Model file for the job. Use its own axes, mm. A direction names the side the tool comes from. Give positions to 0.01 mm unless a question says otherwise; leave off trailing zeros. Order: outer loops, then holes, each group sorted by start corner. A loop starts at its lowest first (then second) coordinate and runs counter-clockwise, first axis right, second up. Notation, with made-up numbers: (-27, 3) - (-17, 3) arc R35 ccw to (-17, 35) - close; hole circle Ø8 at (41, 14). An arc over 180 degrees is marked (long way). Return JSON: item names as keys, results as strings. Group by question number.
Autodesk Inventor part; units mm, degrees
ref_plane "YZ Plane" through (0, 0, 0) normal (1, 0, 0) x (0, 1, 0)
ref_plane "XZ Plane" through (0, 0, 0) normal (0, 1, 0) x (-1, 0, 0)
ref_plane "XY Plane" through (0, 0, 0) normal (0, 0, 1) x (1, 0, 0)
sketch "Sketch1" plane through (0, 0, 0) normal (0, 0, 1) x (1, 0, 0)
  circle A0 centre (0, 0) radius 12.5
  circle A1 centre (0, 0) radius 14.5
  dimension "d0" = 25
  dimension "d1" = 2
extrude "Extrusion1" add sketch "Sketch1" along normal blind 2
sketch "Sketch2" plane through (0, 0, 2) normal (0, 0, 1) x (1, 0, 0)
  circle A0 centre (0, 0) radius 14.5 construction
  line L0 (0, 14.5) -> (0, 0) construction
  line L1 (0, 0) -> (12.5574, -7.25) construction
  line L2 (0, 0) -> (-12.5574, -7.25) construction
  line L3 (0, 0) -> (-12.5574, 7.25) construction
  line L4 (0, 0) -> (12.5574, 7.25) construction
  circle A1 centre (0, 0) radius 14.5
  circle A2 centre (0, 0) radius 12.5
  line L5 (1.3066, 12.4315) -> (1.5157, 14.4206)
  line L6 (-1.3066, 12.4315) -> (-1.5157, 14.4206)
  line L7 (-11.4193, -5.0842) -> (-13.2464, -5.8977)
  line L8 (-10.1127, -7.3473) -> (-11.7307, -8.5229)
  line L9 (10.1127, -7.3473) -> (11.7307, -8.5229)
  line L10 (11.4193, -5.0842) -> (13.2464, -5.8977)
  line L11 (10.1127, 7.3473) -> (11.7307, 8.5229)
  line L12 (11.4193, 5.0842) -> (13.2464, 5.8977)
  line L13 (-11.4193, 5.0842) -> (-13.2464, 5.8977)
  line L14 (-10.1127, 7.3473) -> (-11.7307, 8.5229)
  line L15 (1.3066, -12.4315) -> (1.5157, -14.4206)
  line L16 (-1.3066, -12.4315) -> (-1.5157, -14.4206)
  point P0 (-12.5574, -7.25)
  point P1 (12.5574, -7.25)
  dimension "d4" = 120
  dimension "d5" = 120
  dimension "d6" = 6
  dimension "d7" = 6
  dimension "d10" = 360
  dimension "d14" = 6
  dimension "d15" = 6
  dimension "d18" = 360
extrude "Extrusion2" add sketch "Sketch2" along normal blind 16 contours A1 L9 A2 L10 | L5 A2 L6 A1 | A1 L7 A2 L8
sketch "Sketch3" plane through (0, 0, 2) normal (0, 0, 1) x (1, 0, 0)
  circle A0 centre (0, 0) radius 14.5 construction
  line L0 (0, 14.5) -> (0, 0) construction
  line L1 (0, 0) -> (12.5574, -7.25) construction
  line L2 (0, 0) -> (-12.5574, -7.25) construction
  line L3 (0, 0) -> (-12.5574, 7.25) construction
  line L4 (0, 0) -> (12.5574, 7.25) construction
  circle A1 centre (0, 0) radius 14.5
  circle A2 centre (0, 0) radius 12.5
  line L5 (1.3066, 12.4315) -> (1.5157, 14.4206)
  line L6 (-1.3066, 12.4315) -> (-1.5157, 14.4206)
  line L7 (-11.4193, -5.0842) -> (-13.2464, -5.8977)
  line L8 (-10.1127, -7.3473) -> (-11.7307, -8.5229)
  line L9 (10.1127, -7.3473) -> (11.7307, -8.5229)
  line L10 (11.4193, -5.0842) -> (13.2464, -5.8977)
  line L11 (10.1127, 7.3473) -> (11.7307, 8.5229)
  line L12 (11.4193, 5.0842) -> (13.2464, 5.8977)
  line L13 (-11.4193, 5.0842) -> (-13.2464, 5.8977)
  line L14 (-10.1127, 7.3473) -> (-11.7307, 8.5229)
  line L15 (1.3066, -12.4315) -> (1.5157, -14.4206)
  line L16 (-1.3066, -12.4315) -> (-1.5157, -14.4206)
  point P0 (-12.5574, -7.25)
  point P1 (12.5574, -7.25)
  dimension "d24" = 120
  dimension "d25" = 120
  dimension "d26" = 6
  dimension "d27" = 6
  dimension "d28" = 360
  dimension "d29" = 6
  dimension "d30" = 6
  dimension "d31" = 360
extrude "Extrusion3" cut sketch "Sketch3" against normal blind 1 contours L12 A2 L11 A1 | A1 L16 A2 L15 | L14 A2 L13 A1
fillet "Fillet1" radius 3 6 edges at (1.4111, 13.426, 2) (-1.4111, 13.426, 2) (-12.3329, -5.4909, 2) (12.3329, -5.4909, 2) (-10.9217, -7.9351, 2) (10.9217, -7.9351, 2)
properties part number "_3DPrint"
(1) Pull direction Y, two halves, no side cores. Call faces 4 (the face through (10.91, 7.927, 1.507)), 5 (the face through (-12, -7, 18)), 6 (the face through (-10.91, 7.927, 1.507)), 7 (the face through (12.53, -4.64, 2.9)): released by +Y, released by -Y, zero draft, split by the parting line, or undercut.
(2) Slice it at C-C (z = 13). Give the cut face in (x, y).
(3) Drop flat-ended pins along their axis: pin 1 Ø5 at (x, y) = (7, 11) entering from +Z; pin 2 Ø1.6 at (x, y) = (-12, 7) entering from +Z; pin 3 Ø10 at (y, z) = (8.5, 14.5) entering from -X; pin 4 Ø6 at (y, z) = (6.5, 12) entering from -X. Give the stop position or say it passes through.
(4) Slice it at B-B (x = 0). Give the cut face in (y, z).
(5) Drill centre lines: L1, parallel to Y at x = 0, z = 13.5; L2, parallel to Z at x = 13, y = 2.5; L3, parallel to Z at x = -11, y = 7. Where is each one in solid material? Low to high.
(6) Slice it at A-A (y = 0). Give the cut face in (x, z), and give its area (3 significant figures).
(7) 3-axis set-ups, long thin cutter, end or side, ignore diameter. For faces 1 (the face through (1.41, 13.41, 11.41)), 2 (the face through (-10.91, -7.927, 11.409)), 3 (the face through (-12.32, 5.485, 1.507)): which of +Z, -Z, +X, -X, +Y, -Y reach the whole face in a straight line?
Result set:
{
 "1": {"face 4": "undercut", "face 5": "zero draft", "face 6": "undercut", "face 7": "released by +Y"},
 "2": {"outline": "(-13.25, -5.9) arc R14.5 ccw to (-11.73, -8.52) - (-10.11, -7.35) arc R12.5 cw to (-11.42, -5.08) - close; (-1.52, 14.42) - (-1.31, 12.43) arc R12.5 cw to (1.31, 12.43) - (1.52, 14.42) arc R14.5 ccw to start; (10.11, -7.35) - (11.73, -8.52) arc R14.5 ccw to (13.25, -5.9) - (11.42, -5.08) arc R12.5 cw to start"},
 "3": {"pin 1": "stops at z = 2", "pin 2": "stops at z = 1", "pin 3": "stops at x = -1.42", "pin 4": "passes through"},
 "4": {"outline": "(-14.5, 0) - (-12.5, 0) - (-12.5, 1) - (-14.5, 1) - close; (12.5, 0) - (14.5, 0) - (14.5, 18) - (12.5, 18) - close"},
 "5": {"L1": "y = 12.5 to 14.5", "L2": "z = 0 to 2", "L3": "z = 0 to 1"},
 "6": {"outline": "(-14.5, 0) - (-12.5, 0) - (-12.5, 2) - (-14.5, 2) - close; (12.5, 0) - (14.5, 0) - (14.5, 2) - (12.5, 2) - close", "area": "8.00 mm²"},
 "7": {"face 1": "+Z, +X, -Y", "face 2": "+Z, -Y", "face 3": "+Z"}
}
